Geometry check sheet. Reference: the model listing, model coordinates, mm. A direction names the side the tool comes from. Coordinates: 2 decimals unless noted, no trailing zeros. Write each loop counter-clockwise with the first axis right and the second up, starting at its lowest first coordinate (ties: lowest second). Pieces come first, ordered by that corner, then holes. Notation, with made-up numbers: M -9,66 L 15,66 A29 cw 15,99 Z; hole C 86.5,12 d1. An arc over 180 degrees is marked long. Write each question's results on one line, items separated by ' | '.
Autodesk Inventor part; units mm, degrees
ref_plane "Work Plane1" through (0, 0, 0) normal (0, 0, 1) x (1, 0, 0)
ref_plane "YZ Plane" through (0, 0, 0) normal (1, 0, 0) x (0, 1, 0)
ref_plane "XZ Plane" through (0, 0, 0) normal (0, 1, 0) x (-1, 0, 0)
ref_plane "Work Plane1" through (0, 0, 0) normal (0, 0, 1) x (1, 0, 0)
sketch "base_sketch" plane through (0, 0, 0) normal (0, 0, 1) x (1, 0, 0)
  circle A0 centre (0, -125.6462) radius 1.5
  circle A1 centre (-38, -125.6462) radius 1.5
  line L0 (14.5, -121.6462) -> (-52.5, -121.6462)
  line L1 (-52.5, -121.6462) -> (-52.5, -129.6462)
  line L2 (-52.5, -129.6462) -> (14.5, -129.6462)
  line L3 (14.5, -129.6462) -> (14.5, -121.6462)
  line L4 (-19, -121.6462) -> (-19, -129.6462) construction
  point P0 (0, 0)
  dimension "d1" = 67
  dimension "d4" = 38
  dimension "d5" = 19
  dimension "d6" = 4
  dimension "d7" = 4
extrude "base" add sketch "base_sketch" along normal blind 8
sketch "holes_bolt_head_sketch" plane through (0, 0, 8) normal (0, 0, 1) x (1, 0, 0)
  circle A0 centre (0, -125.6462) radius 1.5 construction
  circle A1 centre (0, -125.6462) radius 2.9
  circle A2 centre (-38, -125.6462) radius 1.5 construction
  circle A3 centre (-38, -125.6462) radius 2.9
  point P0 (0, 0)
  dimension "d10" = 5.8
  dimension "d11" = 5.8
extrude "holes_bolt_head" cut sketch "holes_bolt_head_sketch" against normal blind 3.2
fillet "bolt_head_fillet" radius 0.5 2 edges at (-40.9, -125.6462, 4.8) (-2.9, -125.6462, 4.8)
sketch "walls_sketch" plane through (-52.5, -129.6462, 0) normal (0, -1, 0) x (1, 0, 0)
  line L0 (0, 0) -> (67, 0)
  line L1 (67, 0) -> (67, 8)
  line L2 (0, 8) -> (67, 8)
  line L3 (0, 0) -> (0, 8)
  line L4 (67, 8) -> (0, 8)
  line L5 (0, 8) -> (0, 23.7)
  line L6 (0, 23.7) -> (3, 23.7)
  line L7 (0, 23.7) -> (3, 23.7) construction
  line L8 (3, 23.7) -> (3, 26.3)
  line L9 (3, 26.3) -> (-2.6, 26.3)
  line L10 (-2.6, 26.3) -> (-2.6, 0)
  line L11 (0, 0) -> (67, 0)
  line L12 (-2.6, 0) -> (0, 0)
  line L13 (0, 0) -> (0, 8)
  line L14 (33.5, 8) -> (33.5, 0) construction
  line L15 (67, 8) -> (67, 23.7)
  line L16 (67, 23.7) -> (64, 23.7)
  line L17 (64, 23.7) -> (64, 26.3)
  line L18 (64, 26.3) -> (69.6, 26.3)
  line L19 (69.6, 26.3) -> (69.6, 0)
  line L20 (69.6, 0) -> (67, 0)
  point P0 (52.5, 0)
  dimension "d15" = 15.7
  dimension "d16" = 3
  dimension "d17" = 0
  dimension "d18" = 2.6
  dimension "d19" = 2.6
extrude "walls" add sketch "walls_sketch" against normal up to surface (8 mm away) contours L12 L10 L9 L8 L6 L5 L3 | L1 L15 L16 L17 L18 L19 L20
fillet "wall_top" radius 2 2 edges at (-55.1, -125.6462, 26.3) (17.1, -125.6462, 26.3)
fillet "wall_tooth" radius 1 4 edges at (-49.5, -125.6462, 26.3) (-49.5, -125.6462, 23.7) (11.5, -125.6462, 23.7) (11.5, -125.6462, 26.3)
chamfer "wall_bottom" distance 4 angle 45 2 edges at (17.1, -125.6462, 0) (-55.1, -125.6462, 0)
fillet "wall_bottom_fillet" radius 4 4 edges at (-55.1, -125.6462, 4) (17.1, -125.6462, 4) (13.1, -125.6462, 0) (-51.1, -125.6462, 0)
fillet "inside" radius 0.5 4 edges at (14.5, -125.6462, 8) (-52.5, -125.6462, 8) (-52.5, -125.6462, 23.7) (14.5, -125.6462, 23.7)
equation "\"d5\" = 0.5 * d4"
equation "\"d7\" = d6"
equation "\"d10\" = d11"
properties part number "mount_enclosure_coral_dev_board" material "ABS Plastic"
Q1. Sectioned sample at C-C on z = 3.75. Record the cut outline in (x, y).
Geometry check:
outline: M -54.62,-129.65 L 16.62,-129.65 L 16.62,-121.65 L -54.62,-121.65 Z; hole C -38,-125.65 d3; hole C 0,-125.65 d3
Q2. Sectioned sample at B-B on x = 0. Record the cut outline in (y, z), and give its area (3 significant figures).
Geometry check:
outline: M -129.65,0 L -127.15,0 L -127.15,4.8 L -128.05,4.8 A0.5 cw -128.55,5.3 L -128.55,8 L -129.65,8 Z; M -124.15,0 L -121.65,0 L -121.65,8 L -122.75,8 L -122.75,5.3 A0.5 cw -123.25,4.8 L -124.15,4.8 Z | area: 31.1 mm2
Q3. Mould release check, pull along Z, two halves, no side actions. Record for faces 1 (the cylindrical face through (12.99, -125.59, 0.31)), 2 (the flat face through (-51, -126, 23.7)), 3 (the cylindrical face through (-0.195, -127.133, 2.366)): pulls with the +Z half, pulls with the -Z half, needs draft (parallel to the pull), parting line crosses it, or undercut.
Geometry check:
face 1: pulls with the -Z half | face 2: undercut | face 3: needs draft
Q4. Sectioned sample at D-D on y = -126.5. Give the number of separate pieces and of enclosed holes in the cut face, and give its area (3 significant figures).
Geometry check:
separate pieces: 3 | enclosed holes: 0 | area: 610 mm2
Q5. Scan lines: probe 1 along Y at (x, z) = (0, 2.5); probe 2 along X at (y, z) = (-128.75, 23); probe 3 along X at (y, z) = (-125, 4.5). Record each from-to range of solid material in increasing order.
Geometry check:
probe 1: y = -129.65 to -127.15, -124.15 to -121.65 | probe 2: x = -55.1 to -52.5, 14.5 to 17.1 | probe 3: x = -54.93 to -39.35, -36.65 to -1.35, 1.35 to 16.93
Q6. Access from +Z, -Z, +X, -X, +Y, -Y to the whole of each face (thin tool, end or side, straight path). Record for faces 4 (the cylindrical face through (-0.629, -128.477, 6.669)), 5 (the flat face through (-52.5, -126, 16)), 6 (the flat face through (14, -126, 26.3)).
Geometry check:
face 4: +Z | face 5: +Y, -Y | face 6: +Z, +X, -X, +Y, -Y
Q7. Depth check by flat-ended pin: P1, Ø4, axis at y = -128.5, z = 2.5, coming from the +X side; P2, Ø2.5, axis at x = 0, y = -125.65, coming from the +Z side; P3, Ø1.2, axis at x = 13.5, y = -127.5, coming from the -Z side; P4, Ø0.8, axis at x = -51.5, y = -126, coming from the -Z side. Enter the tip coordinate at first touch or a pass-through.
Geometry check:
P1: stops at x = 16.93 | P2: passes through | P3: stops at z = 0.27 | P4: stops at z = 0.36
Q8. Sectioned sample at A-A on z = 15.75. Record the cut outline in (x, y), and give its area (3 significant figures).
Geometry check:
outline: M -55.1,-129.65 L -52.5,-129.65 L -52.5,-121.65 L -55.1,-121.65 Z; M 14.5,-129.65 L 17.1,-129.65 L 17.1,-121.65 L 14.5,-121.65 Z | area: 41.6 mm2
